Geometry check sheet. Reference: the model listing, model coordinates, mm. Coordinates: 2 decimals unless noted, no trailing zeros. Write each loop counter-clockwise with the first axis right and the second up, starting at its lowest first coordinate (ties: lowest second). Pieces come first, ordered by that corner, then holes. Notation, with made-up numbers: (-20, 23.5) -> (32, 23.5) arc R21 ccw to (32, 55.5) -> close; hole circle Ø8 at (-3.75, 58.25). An arc over 180 degrees is marked (long way). Use a Markdown table: item, result.
```python
from build123d import *

# Parameters (mm, degrees)
SKETCH069_R     = 3
PAD040_DEPTH    = 0.5
SKETCH070_R     = 3
PAD041_DEPTH    = 1.5
SKETCH072_R     = 8
PAD049_DEPTH    = 2
SKETCH071_R     = 2
POCKET046_DEPTH = 4


with BuildPart() as part:
    # Sketch069 → Pad040 (new body)
    with BuildSketch(Plane.XY.offset(32)):
        with Locations((5.5, -22.5)):
            Circle(SKETCH069_R)
    extrude(amount=PAD040_DEPTH)

    # Sketch070 → Pad041 (join)
    with BuildSketch(Plane.XY.offset(32)):
        with Locations((5.5, -22.5)):
            Circle(SKETCH070_R)
    extrude(amount=-PAD041_DEPTH)

    # Sketch072 → Pad049 (join)
    with BuildSketch(Plane.XY.offset(32.5)):
        with Locations((5.5, -22.5)):
            Circle(SKETCH072_R)
    extrude(amount=PAD049_DEPTH)

    # Sketch094 → Revolution (revolve)
    with BuildSketch(Plane(origin=(5.5, -22.5, 18), x_dir=(1, 0, 0), z_dir=(0, -1, 0))):
        with BuildLine():
            Line((0, 18), (0, 16.48024))
            Line((0, 16.48024), (8, 16.48024))
            add(Edge.make_bspline(
                [(0, 18), (2, 18), (5, 19), (8, 16.48024)],
                knots=[0, 0, 0, 0, 1, 1, 1, 1], degree=3))
        make_face()
    revolve(axis=Axis((5.5, -22.5, 18), (0, 0, 1)))

    # Sketch071 (on Face4 of Pad041) → Pocket046 (cut)
    with BuildSketch(Plane(origin=(0, 0, 30.5), x_dir=(1, 0, 0), z_dir=(0, 0, -1))):
        with Locations((5.5, 22.5)):
            Circle(SKETCH071_R)
    extrude(amount=-POCKET046_DEPTH, mode=Mode.SUBTRACT)


solid = part.part
```
Item 1: Section check A-A on z = 33.95. Record the boundary of the cut face in (x, y), then the cut area to 3 significant figures.
Answer block:
| item | result |
|---|---|
| outline | circle Ø16 at (5.5, -22.5); hole circle Ø4 at (5.5, -22.5) |
| area | 188 mm^2 |
Item 2: Thickness scan on L1, parallel to Y at x = 5.5, z = 32.6; L2, parallel to Y at x = 5.5, z = 32.15; L3, parallel to X at y = -22.75, z = 31.15. Record the ranges inside material, lowest first. Write a range as [from, to].
Answer block:
| item | result |
|---|---|
| L1 | y = [-30.5, -24.5], [-20.5, -14.5] |
| L2 | y = [-25.5, -24.5], [-20.5, -19.5] |
| L3 | x = [2.51, 3.52], [7.48, 8.49] |
Item 3: Mould release check, pull along Y, two halves, no side actions. Record for faces 1 (the cylindrical face through (9.19, -29.6, 33.49)), 2 (the flat face through (3, -22, 30.5)), 3 (the cylindrical face through (3.9, -21.3, 32.5)): +Y half, -Y half, draft (parallel to the pull), parting line (faces both ways), or undercut.
Answer block:
| item | result |
|---|---|
| face 1 | parting line |
| face 2 | draft |
| face 3 | undercut |
Item 4: Depth check by flat-ended pin: P1, Ø2, axis at y = -18.5, z = 32, coming from the -X side; P2, Ø8, axis at x = 6.5, y = -19.5, coming from the -Z side; P3, Ø3.5, axis at x = 5.5, y = -22.5, coming from the -Z side; P4, Ø3, axis at x = 7.5, z = 33, coming from the -Y side. Enter the tip coordinate at first touch or a pass-through.
Answer block:
| item | result |
|---|---|
| P1 | stops at x = -1.86 |
| P2 | stops at z = 30.5 |
| P3 | stops at z = 34.5 |
| P4 | stops at y = -30.48 |
